Can you work these out from the model? Positions are in its coordinate system, mm. A direction names the side the tool comes from. Give positions to 0.01 mm unless a question says otherwise; leave off trailing zeros. Write each loop counter-clockwise with the first axis right and the second up, starting at its lowest first coordinate (ties: lowest second). Pieces come first, ordered by that corner, then holes. Notation, with made-up numbers: (-10, 14.25) - (26, 14.25) arc R14 ccw to (26, 33.25) - close; hole circle Ø4 at (13, -7). An arc over 180 degrees is marked (long way). Use a Markdown table: item, result. Add a question column.
```python
from build123d import *

# Parameters (mm, degrees)
SCHIZZO1_W                   = 20
SCHIZZO1_H                   = 1.5
SCHIZZO3_R                   = 3
ESTRUSIONE_ESTRUSIONE1_DEPTH = 2
SCHIZZO4_W                   = 7
SCHIZZO4_H                   = 1
TAGLIO_ESTRUSIONE1_DEPTH     = 0.7
RACCORDO1_R                  = 0.7


with BuildPart() as part:
    # Schizzo1 → Rivoluzione-Sottile1 (revolve)
    with BuildSketch(Plane.XY):
        with Locations((-10, -0.75)):
            Rectangle(SCHIZZO1_W, SCHIZZO1_H)
    revolve(axis=Axis((0, 0, 0), (-1, 0, 0)))

    # Schizzo3 → Estrusione-Estrusione1 (add)
    with BuildSketch(Plane(origin=(0, 0, 0), x_dir=(0, 0, -1), z_dir=(1, 0, 0))):
        Circle(SCHIZZO3_R)
    extrude(amount=ESTRUSIONE_ESTRUSIONE1_DEPTH)

    # Schizzo4 → Taglio-Estrusione1 (cut)
    with BuildSketch(Plane(origin=(2, 0, 0), x_dir=(0, 0, -1), z_dir=(1, 0, 0))):
        Rectangle(SCHIZZO4_W, SCHIZZO4_H)
    extrude(amount=-TAGLIO_ESTRUSIONE1_DEPTH, mode=Mode.SUBTRACT)

    # Raccordo1
    raccordo1_edges = [part.edges().sort_by_distance(p)[0] for p in [
        (2, -3, 0),
        (2, 3, 0),
    ]]
    fillet(raccordo1_edges, radius=RACCORDO1_R)


solid = part.part
```
Q1. Suppose I cut it at C-C (x = -6.5). Please give me the cut outline in (y, z), and give its area (3 significant figures).
Q2. If I drill on probe 1 along X at (y, z) = (1, 2); probe 2 along Y at (x, z) = (-11, 0.1); probe 3 along Z at (x, y) = (-13.5, -0.25), over which ranges is the centre line in solid material (lowest first)? Write a range as [from, to].
Q3. I'm going to push flat-ended pins straight in: P1, Ø3, axis at x = -12.5, y = 0, coming from the -Z side; P2, Ø1.1, axis at y = 0, z = -1.5, coming from the +X side; P3, Ø1.5, axis at x = -1.5, y = -1.5, coming from the +Z side; P4, Ø2, axis at x = -2.5, z = -1.5, coming from the +Y side. Where does each tip first touch, or does it pass through?
Q4. On a 3-axis mill with a long thin cutter (end or side, diameter ignored), from which of +Z, -Z, +X, -X, +Y, -Y can I reach the whole of each face in a straight line? I mean faces 4 (the flat face through (2, -1, 0)), 5 (the flat face through (0, -1.3, -1.3)). Say none if no direction works.
Q5. Suppose I cut it at B-B (z = 0). Please give me the cut outline in (x, y), and give its area (3 significant figures).
Q6. Suppose I cut it at A-A (y = 0). Please give me the cut outline in (x, z).
Q7. If we mould it in two halves opening along Y, with no side actions, what happens to faces 1 (the cylindrical face through (1, 0, 3)), 2 (the flat face through (2, 1, 0)), 3 (the flat face through (1.3, 0, 0))? For each: released by +Y, released by -Y, zero draft, split by the parting line, or undercut.
Derived:
| question | item | result |
|---|---|---|
| 1 | outline | circle Ø3 at (0, 0) |
| 1 | area | 7.07 mm² |
| 2 | probe 1 | [0, 2] |
| 2 | probe 2 | [-1.5, 1.5] |
| 2 | probe 3 | [-1.48, 1.48] |
| 3 | P1 | z = -1.5 |
| 3 | P2 | x = 2 |
| 3 | P3 | z = 1.3 |
| 3 | P4 | y = 1.41 |
| 4 | face 4 | +Z, -Z, +X, +Y, -Y |
| 4 | face 5 | -X |
| 5 | outline | (-20, -1.5) - (0, -1.5) - (0, -3) - (1.3, -3) arc R0.7 ccw to (2, -2.3) - (2, -0.5) - (1.3, -0.5) - (1.3, 0.5) - (2, 0.5) - (2, 2.3) arc R0.7 ccw to (1.3, 3) - (0, 3) - (0, 1.5) - (-20, 1.5) - close |
| 5 | area | 71.1 mm² |
| 6 | outline | (-20, -1.5) - (0, -1.5) - (0, -3) - (1.3, -3) - (1.3, 3) - (0, 3) - (0, 1.5) - (-20, 1.5) - close |
| 7 | face 1 | split by the parting line |
| 7 | face 2 | zero draft |
| 7 | face 3 | undercut |
